Work out the finished part from the listing and answer in its coordinate system (mm). Face numbers are marked on the shaded views. A direction names the side the tool comes from. Coordinates: 2 decimals unless noted, no trailing zeros. Write each loop counter-clockwise with the first axis right and the second up, starting at its lowest first coordinate (ties: lowest second). Pieces come first, ordered by that corner, then holes. Notation, with made-up numbers: (41, 60.25) - (88, 60.25) arc R28 ccw to (88, 91.25) - close; hole circle Ø9 at (49, -39.5). An arc over 180 degrees is marked (long way). Use a Markdown table: item, result. Add a question column.
(1) The part is cut by section A-A, the plane z = 10.5. Give the vertices of the cut face in (x, y) (3 decimals), then the cut area to 3 significant figures.
(2) A tool of negligible diameter and unlimited length cuts with its end or side. For the marked faces 1, 2, 3 and 4, from which of +Z, -Z, +X, -X, +Y, -Y can it reach the whole face along a straight path? Write none if from no direction.
(3) The part is cut by section B-B, the plane z = -5. Give the vertices of the cut face in (x, y) (3 decimals).
(4) The part is cut by section C-C, the plane y = 2.5. Give the vertices of the cut face in (x, z) (3 decimals).
(5) The part is cut by section D-D, the plane x = -12. Give the vertices of the cut face in (y, z).
(6) Find the intervals of material crossed by line 1 (X direction, y = 5.25, z = -5) (3 decimals); line 2 (Z direction, x = -25, y = 4); line 3 (X direction, y = 5, z = -2.5) (3 decimals), in increasing order. Write a range as from..to.
(7) Given pin 1 Ø2 at (x, z) = (-24.5, 5) entering from +Y; pin 2 Ø3 at (y, z) = (1.5, -18.5) entering from -X; pin 3 Ø3 at (x, y) = (33.5, 1.5) entering from -Z; pin 4 Ø1.9 at (x, y) = (-7, 4.5) entering from +Z, each flat-ended and moving along its own axis, determine where each tip first touches the part or whether it passes through.
from build123d import *

# Parameters (mm, degrees)
SKETCH1_R           = 1.70053
SKETCH1_W           = 41.91
SKETCH1_H           = 21.844
BOSS_EXTRUDE1_DEPTH = 6.35
CUT_EXTRUDE1_DEPTH  = 50.192057177


with BuildPart() as part:
    # Sketch1 → Boss-Extrude1 (new body)
    with BuildSketch(Plane(origin=(0, 0, 0), x_dir=(1, 0, 0), z_dir=(0, 1, 0))):
        Polygon((-6.35, 25.4), (6.35, 25.4), (28.94584, 25.4), (28.94584, 12.7), (41.64584, 12.7), (41.64584, -12.7), (28.94584, -12.7), (28.94584, -25.4), (6.35, -25.4), (-6.35, -25.4), (-28.94584, -25.4), (-28.94584, -12.7), (-41.64584, -12.7), (-41.64584, 12.7), (-28.94584, 12.7), (-28.94584, 25.4), align=None)
        with Locations(Location((-24.49957, 5, 0), (0, 0, 270))):
            Circle(SKETCH1_R, mode=Mode.SUBTRACT)
        with Locations(Location((-24.49957, -5, 0), (0, 0, 270))):
            Circle(SKETCH1_R, mode=Mode.SUBTRACT)
        with Locations(Location((24.49957, -5, 0), (0, 0, 270))):
            Circle(SKETCH1_R, mode=Mode.SUBTRACT)
        with Locations(Location((24.49957, 5, 0), (0, 0, 270))):
            Circle(SKETCH1_R, mode=Mode.SUBTRACT)
        Rectangle(SKETCH1_W, SKETCH1_H, mode=Mode.SUBTRACT)
    extrude(amount=BOSS_EXTRUDE1_DEPTH)

    # Sketch2 → Cut-Extrude1 (cut, through all)
    with BuildSketch(Plane(origin=(0, 6.35, 0), x_dir=(1, 0, 0), z_dir=(0, 1, 0))):
        Polygon((-28.94584, -12.7), (-20.955, -12.7), (-20.955, -10.922), (20.955, -10.922), (20.955, -12.7), (28.94584, -12.7), (28.94584, -25.4), (-28.94584, -25.4), align=None)
    extrude(amount=-CUT_EXTRUDE1_DEPTH, mode=Mode.SUBTRACT)


solid = part.part
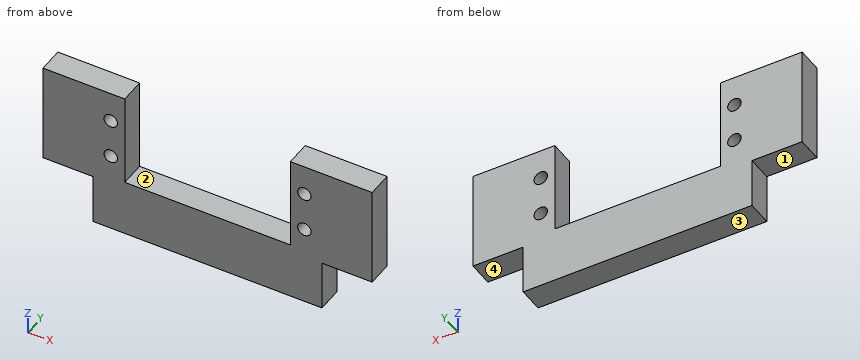
Model answer:
| question | item | result |
|---|---|---|
| 1 | outline | (-41.646, 0) - (-20.955, 0) - (-20.955, 6.35) - (-41.646, 6.35) - close; (20.955, 0) - (41.646, 0) - (41.646, 6.35) - (20.955, 6.35) - close |
| 1 | area | 263 mm^2 |
| 2 | face 1 | -Z, -X, +Y, -Y |
| 2 | face 2 | +Z, +Y, -Y |
| 2 | face 3 | -Z, +X, -X, +Y, -Y |
| 2 | face 4 | -Z, +X, +Y, -Y |
| 3 | outline | (-41.646, 0) - (-26.2, 0) - (-26.2, 6.35) - (-41.646, 6.35) - close; (-22.799, 0) - (-20.955, 0) - (-20.955, 6.35) - (-22.799, 6.35) - close; (20.955, 0) - (22.799, 0) - (22.799, 6.35) - (20.955, 6.35) - close; (26.2, 0) - (41.646, 0) - (41.646, 6.35) - (26.2, 6.35) - close |
| 4 | outline | (-41.646, -12.7) - (-28.946, -12.7) - (-28.946, -25.4) - (28.946, -25.4) - (28.946, -12.7) - (41.646, -12.7) - (41.646, 12.7) - (20.955, 12.7) - (20.955, -10.922) - (-20.955, -10.922) - (-20.955, 12.7) - (-41.646, 12.7) - close; hole circle Ø3.401 at (-24.5, -5); hole circle Ø3.401 at (-24.5, 5); hole circle Ø3.401 at (24.5, -5); hole circle Ø3.401 at (24.5, 5) |
| 5 | outline | (0, -25.4) - (6.35, -25.4) - (6.35, -10.92) - (0, -10.92) - close |
| 6 | line 1 | -41.646..-26.2, -22.799..-20.955, 20.955..22.799, 26.2..41.646 |
| 6 | line 2 | -25.4..-6.63, -3.37..3.37, 6.63..12.7 |
| 6 | line 3 | -41.646..-20.955, 20.955..41.646 |
| 7 | pin 1 | through |
| 7 | pin 2 | x = -28.95 |
| 7 | pin 3 | z = -12.7 |
| 7 | pin 4 | z = -10.92 |
